```python
from build123d import *

# Parameters (mm, degrees)
F1_DEPTH = 38.1
F2_R     = 5.08
F3_R     = 12.7
F4_DEPTH = 38.1


with BuildPart() as f1:
    # F0 (on Front) → F1 (new body)
    with BuildSketch(Plane.XZ):
        with BuildLine():
            Line((-25.4, 93.829548), (-25.4, 74.779548))
            Line((-25.4, 74.779548), (101.6, 74.779548))
            Line((101.6, 74.779548), (101.6, 93.829548))
            Line((101.6, 93.829548), (76.2, 93.829548))
            Line((76.2, 93.829548), (76.2, 106.529548))
            ThreePointArc((76.2, 106.529548), (38.1, 144.629548), (0, 106.529548))
            Line((0, 106.529548), (0, 93.829548))
            Line((0, 93.829548), (-25.4, 93.829548))
        make_face()
    extrude(amount=F1_DEPTH)

    # F2
    f2_edges = [f1.edges().sort_by_distance(p)[0] for p in [
        (38.1, -38.1, 144.629548),
        (38.1, 0, 144.629548),
        (88.9, -38.1, 93.829548),
        (101.6, -19.05, 93.829548),
        (88.9, 0, 93.829548),
        (-12.7, -38.1, 93.829548),
        (-12.7, 0, 93.829548),
        (-25.4, -19.05, 93.829548),
    ]]
    fillet(f2_edges, radius=F2_R)

    # F3 (on face) → F4 (cut)
    with BuildSketch(Plane.XZ.offset(38.1)):
        with Locations((38.1, 106.529548)):
            Circle(F3_R)
    extrude(amount=-F4_DEPTH, mode=Mode.SUBTRACT)


solid = f1.part
```
Model file for the job. Use its own axes, mm. A direction names the side the tool comes from. Coordinates: 2 decimals unless noted, no trailing zeros. Loops run counter-clockwise (first coordinate to the right, second up) from the corner with the lowest first, then second, coordinate; pieces in that order, holes last. Notation, with made-up numbers: (59, -8.5) -> (101, -8.5) arc R18 cw to (101, 9.5) -> close; hole circle Ø1 at (23, -22.75). An arc over 180 degrees is marked (long way). Answer as a JSON object with one key per item and string values.
Q1. Pull direction Z, two halves, no side cores. Call faces 5 (the flat face through (37, -19, 74.78)), 6 (the cylindrical face through (44.927, -19.317, 117.238)), 7 (the cylindrical face through (-10.373, -36.572, 92.381)): released by +Z, released by -Z, zero draft, split by the parting line, or undercut.
Report:
{"face 5": "released by -Z", "face 6": "undercut", "face 7": "released by +Z"}
Q2. 3-axis set-ups, long thin cutter, end or side, ignore diameter. For faces 1 (the cylindrical face through (74.751, -36.572, 99.74)), 2 (the cylindrical face through (86.147, -1.528, 92.381)), 3 (the flat face through (0, -19, 100)), 4 (the flat face through (76.2, -19, 100)): which of +Z, -Z, +X, -X, +Y, -Y reach the whole face in a straight line?
Report:
{"face 1": "+Z, +X, -Y", "face 2": "+Z, +X, +Y", "face 3": "+Z, -X, +Y, -Y", "face 4": "+Z, +X, +Y, -Y"}
Q3. Flat gauge pins, fed straight in: P1, Ø4, axis at x = 43, y = -20, coming from the +Z side; P2, Ø4, axis at x = 70, z = 119, coming from the +Y side; P3, Ø16.5, axis at x = 87.5, y = -16, coming from the +Z side; P4, Ø6.5, axis at y = -25.5, z = 103, coming from the -X side. Where does each tip first touch, or does it go through?
Report:
{"P1": "stops at z = 144.52", "P2": "stops at y = 0", "P3": "stops at z = 93.83", "P4": "stops at x = 0"}
Q4. Cut at B-B (x = 38.1). List the corners of the cut face in (y, z), and give its area (3 significant figures).
Report:
{"outline": "(-38.1, 74.78) -> (0, 74.78) -> (0, 93.83) -> (-38.1, 93.83) -> close; (-38.1, 119.23) -> (0, 119.23) -> (0, 139.55) arc R5.08 ccw to (-5.08, 144.63) -> (-33.02, 144.63) arc R5.08 ccw to (-38.1, 139.55) -> close", "area": "1,680 mm2"}
Q5. Cut at C-C (z = 102). List the corners of the cut face in (x, y), and give its area (3 significant figures).
Report:
{"outline": "(0, -33.02) arc R5.08 ccw to (5.08, -38.1) -> (26.24, -38.1) -> (26.24, 0) -> (5.08, 0) arc R5.08 ccw to (0, -5.08) -> close; (49.96, -38.1) -> (71.12, -38.1) arc R5.08 ccw to (76.2, -33.02) -> (76.2, -5.08) arc R5.08 ccw to (71.12, 0) -> (49.96, 0) -> close", "area": "1,980 mm2"}
Q6. Cut at A-A (y = -22). List the corners of the cut face in (x, z), and give its area (3 significant figures).
Report:
{"outline": "(-25.4, 74.78) -> (101.6, 74.78) -> (101.6, 88.75) arc R5.08 ccw to (96.52, 93.83) -> (76.2, 93.83) -> (76.2, 106.53) arc R38.1 ccw to (0, 106.53) -> (0, 93.83) -> (-20.32, 93.83) arc R5.08 ccw to (-25.4, 88.75) -> close; hole circle Ø25.4 at (38.1, 106.53)", "area": "5,150 mm2"}
Q7. Probe probe 1 along Z at (x, y) = (38, -9); probe 2 along X at (y, z) = (-13, 108.5); probe 3 along X at (y, z) = (-22.5, 104). List the from-to ranges inside material, lowest first.
Report:
{"probe 1": "z = 74.78 to 93.83, 119.23 to 144.63", "probe 2": "x = 0.05 to 25.55, 50.65 to 76.15", "probe 3": "x = 0 to 25.65, 50.55 to 76.2"}
Q8. Cut at D-D (y = -35.5). List the corners of the cut face in (x, z).
Report:
{"outline": "(-25.4, 74.78) -> (101.6, 74.78) -> (101.6, 88.75) arc R5.08 ccw to (99, 93.18) -> (75.55, 93.18) -> (75.55, 106.53) arc R37.45 ccw to (0.65, 106.53) -> (0.65, 93.18) -> (-22.8, 93.18) arc R5.08 ccw to (-25.4, 88.75) -> close; hole circle Ø25.4 at (38.1, 106.53)"}
